Source: three-view drawing plus pictorial views. Frame: mm from the lowest corner of the part. Round coordinates to 2 decimals unless told otherwise and drop trailing zeros. Loops run counter-clockwise (first coordinate to the right, second up) from the corner with the lowest first, then second, coordinate; pieces in that order, holes last. Notation, with made-up numbers: (-20.5, 1) -> (-12.5, 1) arc R9 ccw to (-12.5, 8) -> close; hole circle Ø11 at (66, -8.75). An arc over 180 degrees is marked (long way). Answer in a Markdown table with one row per item. Add a question column.
Q1. Pin query (flat end, axial travel): pin 1 (2 mm diameter, centred on x = 18, y = 29.5, fed in from -Z); pin 2 (3.5 mm diameter, centred on x = 26.67, y = 5.08, fed in from -Z) (3 decimals); pin 3 (3 mm diameter, centred on y = 21, z = 2, fed in from +X); pin 4 (0.8 mm diameter, centred on y = 18.5, z = 2, fed in from -X). Return the tip coordinate at first contact, or that it passes through.
Q2. Section B-B, the plane z = 5.08. Output: boundary loops of the cut face in (x, y).
Q3. Section D-D, the plane x = 26.67. Output: boundary loops of the cut face in (y, z) (3 decimals).
Q4. Ray query, L1, parallel to X at y = 1.7, z = 5.08; L2, parallel to Y at x = 26.67, z = 1.9 (3 decimals); L3, parallel to Y at x = 11.43, z = 1.35 (3 decimals). Return the intervals inside material, ascending. Write a range as from..to.
Q5. Section A-A, the plane x = 11.43. Output: boundary loops of the cut face in (y, z) (3 decimals).
Q6. Mould query, pull axis X, two halves, no side actions, for the marked faces 1 and 2. Classes: pulls with the +X half, pulls with the -X half, needs draft (parallel to the pull), parting line crosses it, or undercut.
Q7. Section C-C, the plane y = 33.02. Output: boundary loops of the cut face in (x, z) (3 decimals), and give its area (3 significant figures).
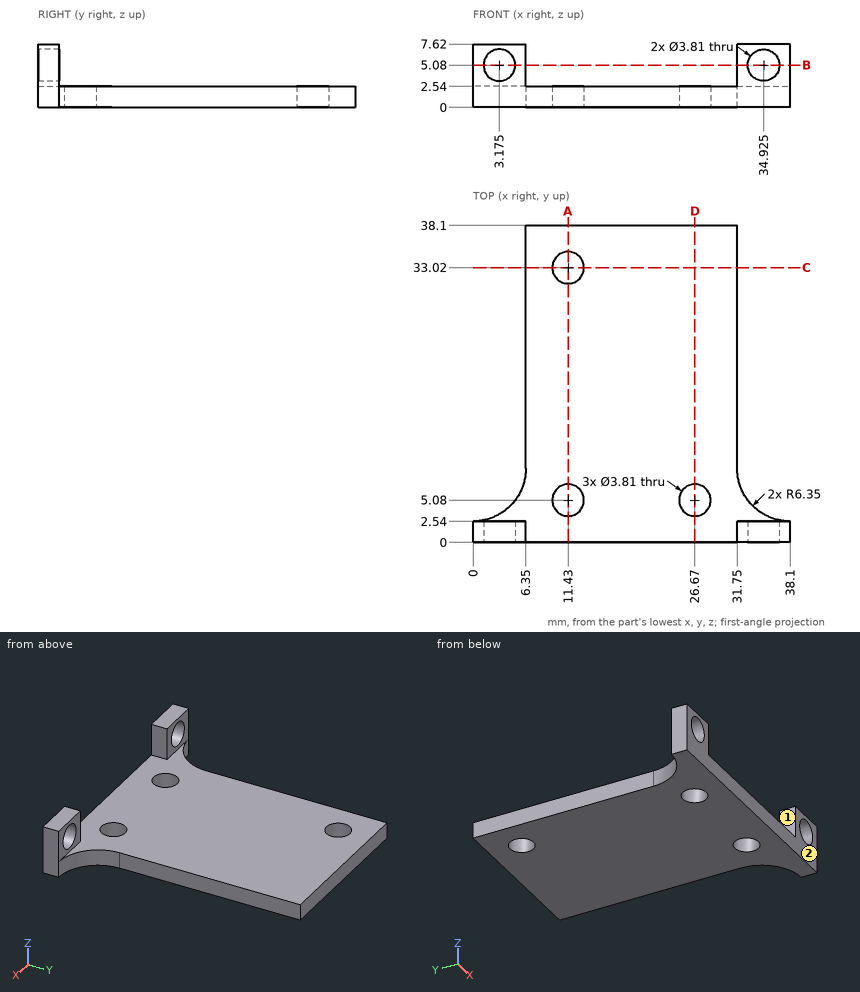
Answer block:
| question | item | result |
|---|---|---|
| 1 | pin 1 | z = 0 |
| 1 | pin 2 | through |
| 1 | pin 3 | x = 31.75 |
| 1 | pin 4 | x = 6.35 |
| 2 | outline | (0, 0) -> (1.27, 0) -> (1.27, 2.54) -> (0, 2.54) -> close; (5.08, 0) -> (6.35, 0) -> (6.35, 2.54) -> (5.08, 2.54) -> close; (31.75, 0) -> (33.02, 0) -> (33.02, 2.54) -> (31.75, 2.54) -> close; (36.83, 0) -> (38.1, 0) -> (38.1, 2.54) -> (36.83, 2.54) -> close |
| 3 | outline | (0, 0) -> (3.175, 0) -> (3.175, 2.54) -> (0, 2.54) -> close; (6.985, 0) -> (38.1, 0) -> (38.1, 2.54) -> (6.985, 2.54) -> close |
| 4 | L1 | 0..1.27, 5.08..6.35, 31.75..33.02, 36.83..38.1 |
| 4 | L2 | 0..3.175, 6.985..38.1 |
| 4 | L3 | 0..3.175, 6.985..31.115, 34.925..38.1 |
| 5 | outline | (0, 0) -> (3.175, 0) -> (3.175, 2.54) -> (0, 2.54) -> close; (6.985, 0) -> (31.115, 0) -> (31.115, 2.54) -> (6.985, 2.54) -> close; (34.925, 0) -> (38.1, 0) -> (38.1, 2.54) -> (34.925, 2.54) -> close |
| 6 | face 1 | undercut |
| 6 | face 2 | needs draft |
| 7 | outline | (6.35, 0) -> (9.525, 0) -> (9.525, 2.54) -> (6.35, 2.54) -> close; (13.335, 0) -> (31.75, 0) -> (31.75, 2.54) -> (13.335, 2.54) -> close |
| 7 | area | 54.8 mm^2 |
